Geometry: final body of the model. Coordinates: model frame, mm. A direction names the side the tool comes from. Give positions to 0.01 mm unless a question says otherwise; leave off trailing zeros. Answer as a JSON object with one key per item and string values.
from build123d import *

# Parameters (mm, degrees)
ESQUISSE1_R        = 1.5
ESQUISSE1_W        = 4
ESQUISSE1_H        = 1.5
ESQUISSE1_W_2      = 5
ESQUISSE1_H_2      = 5
BOSS_EXTRU_1_DEPTH = 5
SKETCH1_W          = 40
SKETCH1_H          = 20
SKETCH1_W_2        = 10
SKETCH1_H_2        = 10
CUT_EXTRUDE1_DEPTH = 10
FILLET2_R          = 10
FILLET3_R          = 2


with BuildPart() as part:
    # Esquisse1 → Boss.-Extru.1 (new body)
    with BuildSketch(Plane.XY):
        Polygon((0, 35), (0, 15), (5, 15), (5, 1.5), (7, 1.5), (7, 2.6), (9.3, 2.6), (9.3, 1.5), (15, 1.5), (15, -1.5), (9.3, -1.5), (9.3, -2.6), (7, -2.6), (7, -1.5), (5, -1.5), (5, -15), (0, -15), (0, -35), (5, -35), (5, -40), (233, -40), (233, -35), (238, -35), (238, -15), (233, -15), (233, -1.5), (231, -1.5), (231, -2.6), (228.7, -2.6), (228.7, -1.5), (223, -1.5), (223, 1.5), (228.7, 1.5), (228.7, 2.6), (231, 2.6), (231, 1.5), (233, 1.5), (233, 15), (238, 15), (238, 35), (233, 35), (233, 40), (5, 40), (5, 35), align=None)
        with Locations((223, 27.5)):
            Circle(ESQUISSE1_R, mode=Mode.SUBTRACT)
        with Locations((223, -27.5)):
            Circle(ESQUISSE1_R, mode=Mode.SUBTRACT)
        with Locations((67, -27.5)):
            Circle(ESQUISSE1_R, mode=Mode.SUBTRACT)
        with Locations((67, 27.5)):
            Circle(ESQUISSE1_R, mode=Mode.SUBTRACT)
        with Locations((183, -34.25)):
            Circle(ESQUISSE1_R, mode=Mode.SUBTRACT)
        with Locations(Location((183, 34.25, 0), (0, 0, 90))):
            Circle(ESQUISSE1_R, mode=Mode.SUBTRACT)
        with Locations(Location((103, 34.25, 0), (0, 0, 90))):
            Circle(ESQUISSE1_R, mode=Mode.SUBTRACT)
        with Locations((103, -34.25)):
            Circle(ESQUISSE1_R, mode=Mode.SUBTRACT)
        with Locations((34, -10.75)):
            Rectangle(ESQUISSE1_W, ESQUISSE1_H, mode=Mode.SUBTRACT)
        with Locations((34, 10.75)):
            Rectangle(ESQUISSE1_W, ESQUISSE1_H, mode=Mode.SUBTRACT)
        with Locations((53, 10.75)):
            Rectangle(ESQUISSE1_W, ESQUISSE1_H, mode=Mode.SUBTRACT)
        with Locations((53, -10.75)):
            Rectangle(ESQUISSE1_W, ESQUISSE1_H, mode=Mode.SUBTRACT)
        with Locations((215.5, 27.5)):
            Rectangle(ESQUISSE1_W_2, ESQUISSE1_H_2, mode=Mode.SUBTRACT)
        with Locations((230.5, 27.5)):
            Rectangle(ESQUISSE1_W_2, ESQUISSE1_H_2, mode=Mode.SUBTRACT)
        with Locations((215.5, -27.5)):
            Rectangle(ESQUISSE1_W_2, ESQUISSE1_H_2, mode=Mode.SUBTRACT)
        with Locations((230.5, -27.5)):
            Rectangle(ESQUISSE1_W_2, ESQUISSE1_H_2, mode=Mode.SUBTRACT)
        with Locations((59.5, -27.5)):
            Rectangle(ESQUISSE1_W_2, ESQUISSE1_H_2, mode=Mode.SUBTRACT)
        with Locations((74.5, -27.5)):
            Rectangle(ESQUISSE1_W_2, ESQUISSE1_H_2, mode=Mode.SUBTRACT)
        with Locations((59.5, 27.5)):
            Rectangle(ESQUISSE1_W_2, ESQUISSE1_H_2, mode=Mode.SUBTRACT)
        with Locations((74.5, 27.5)):
            Rectangle(ESQUISSE1_W_2, ESQUISSE1_H_2, mode=Mode.SUBTRACT)
        with Locations((175.5, -34.25)):
            Rectangle(ESQUISSE1_W_2, ESQUISSE1_H_2, mode=Mode.SUBTRACT)
        with Locations((190.5, -34.25)):
            Rectangle(ESQUISSE1_W_2, ESQUISSE1_H_2, mode=Mode.SUBTRACT)
        with Locations((175.5, 34.25)):
            Rectangle(ESQUISSE1_W_2, ESQUISSE1_H_2, mode=Mode.SUBTRACT)
        with Locations((190.5, 34.25)):
            Rectangle(ESQUISSE1_W_2, ESQUISSE1_H_2, mode=Mode.SUBTRACT)
        with Locations((95.5, 34.25)):
            Rectangle(ESQUISSE1_W_2, ESQUISSE1_H_2, mode=Mode.SUBTRACT)
        with Locations((110.5, 34.25)):
            Rectangle(ESQUISSE1_W_2, ESQUISSE1_H_2, mode=Mode.SUBTRACT)
        with Locations((95.5, -34.25)):
            Rectangle(ESQUISSE1_W_2, ESQUISSE1_H_2, mode=Mode.SUBTRACT)
        with Locations((110.5, -34.25)):
            Rectangle(ESQUISSE1_W_2, ESQUISSE1_H_2, mode=Mode.SUBTRACT)
    extrude(amount=BOSS_EXTRU_1_DEPTH)

    # Sketch1 → Cut-Extrude1 (cut)
    with BuildSketch(Plane(origin=(0, 0, 0), x_dir=(-1, 0, 0), z_dir=(0, 0, -1))):
        with Locations((-102, 30)):
            Rectangle(SKETCH1_W, SKETCH1_H)
        with Locations((-183, 0)):
            Rectangle(SKETCH1_W_2, SKETCH1_H_2)
    extrude(amount=-CUT_EXTRUDE1_DEPTH, mode=Mode.SUBTRACT)

    # Fillet2
    fillet2_edges = [part.edges().sort_by_distance(p)[0] for p in [
        (122, 20, 2.5),
        (82, 20, 2.5),
    ]]
    fillet(fillet2_edges, radius=FILLET2_R)
    fillet2_2_edges = [part.edges().sort_by_distance(p)[0] for p in [
        (122, 40, 2.5),
        (82, 40, 2.5),
    ]]
    fillet(fillet2_2_edges, radius=FILLET2_R - 0.0001)  # a hair under: the kernel refuses the full size

    # Fillet3
    fillet3_edges = [part.edges().sort_by_distance(p)[0] for p in [
        (188, -5, 2.5),
        (188, 5, 2.5),
        (178, 5, 2.5),
        (178, -5, 2.5),
    ]]
    fillet(fillet3_edges, radius=FILLET3_R)


solid = part.part
1) Line query: line 1 (Y direction, x = 103, z = 3.6); line 2 (Y direction, x = 186, z = 1.75); line 3 (X direction, y = 34.25, z = 2.8). Output: solid intervals per line, ascending. Write a range as from..to.
Geometry check:
{"line 1": "y = -40..-35.75, -32.75..20", "line 2": "y = -40..-5, 5..40", "line 3": "x = 0..81.05, 122.95..173, 178..181.5, 184.5..188, 193..238"}
2) Cut plane A-A on z = 1.5. Give the number of separate pieces and of enclosed holes in the cut face, and give its area (3 significant figures).
Geometry check:
{"separate pieces": "1", "enclosed holes": "26", "area": "17,200 mm2"}
3) Pull-direction query (Y, two-part tool) for faces 3 (the flat face through (53, -10, 2)), 4 (the flat face through (183, 40, 2)), 5 (the flat face through (238, -25, 2)); classes: pulls with the +Y half, pulls with the -Y half, needs draft (parallel to the pull), parting line crosses it, or undercut.
Geometry check:
{"face 3": "undercut", "face 4": "pulls with the +Y half", "face 5": "needs draft"}
4) Set-up query: faces 1 (the flat face through (175, 36.75, 2)), 2 (the cylindrical face through (84.85, 23.01, 2.54)). Return all of +Z, -Z, +X, -X, +Y, -Y with unobstructed straight access to the full face (end or side cutting, diameter ignored); none if empty.
Geometry check:
{"face 1": "+Z, -Z", "face 2": "+Z, -Z, +Y"}
5) Contact query for flat-ended pins moving along their axis: P1, Ø3, axis at x = 128, z = 2, coming from the +Y side; P2, Ø1.5, axis at y = 38, z = 2, coming from the +X side. Output: stop coordinate, or through.
Geometry check:
{"P1": "stops at y = 39.68", "P2": "stops at x = 233"}
